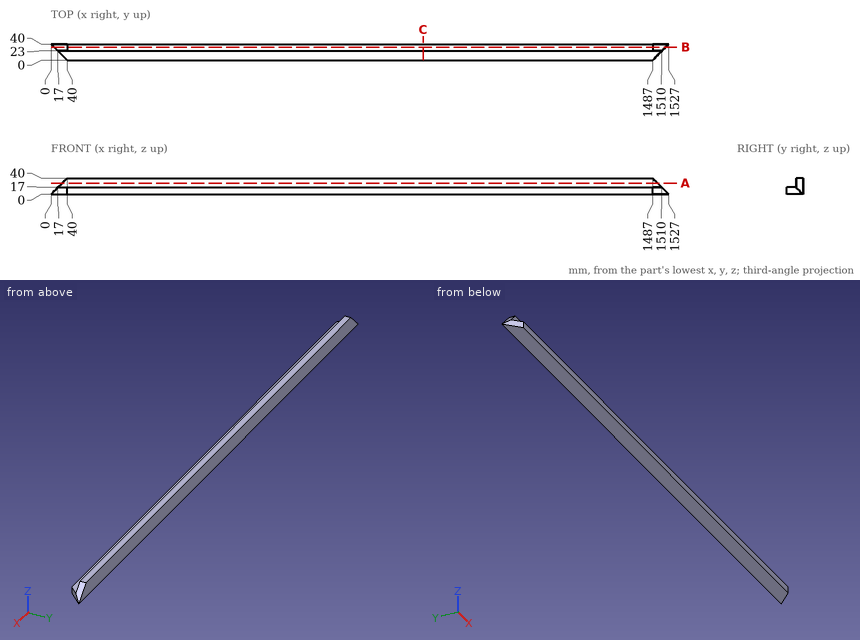
Check sheet for the drawn part. Datum: minimum x, y, z corner. Units: mm. Round coordinates to 2 decimals unless told otherwise and drop trailing zeros. Loops run counter-clockwise (first coordinate to the right, second up) from the corner with the lowest first, then second, coordinate; pieces in that order, holes last.
Item 1: Cross-section at B-B on y = 32.5. Record the boundary of the cut face in (x, z).
Item 2: Thickness scan on line 1 (Z direction, x = 881, y = 16); line 2 (Y direction, x = 729, z = 36); line 3 (X direction, y = 2, z = 7). Record the ranges inside material, lowest first.
Item 3: Cross-section at C-C on x = 919.5. Record the boundary of the cut face in (y, z), then the cut area to 3 significant figures.
Item 4: Cross-section at A-A on z = 28. Record the boundary of the cut face in (x, y).
Item 5: Gauge pin test, flat ends, axial feed: pin 1 (1 mm diameter, centred on y = 27.5, z = 8, fed in from -X); pin 2 (1 mm diameter, centred on y = 24, z = 34.5, fed in from +X); pin 3 (8 mm diameter, centred on x = 259, z = 22, fed in from -Y). Record the tip position at first contact, or that the pin passes through.
Answer sheet:
1. outline: (7.5, 0) - (1519.5, 0) - (1519.5, 7.5) - (1487, 40) - (40, 40) - (7.5, 7.5) - close
2. line 1: z = 0 to 17
2. line 2: y = 23 to 40
2. line 3: x = 38 to 1489
3. outline: (0, 0) - (40, 0) - (40, 40) - (23, 40) - (23, 17) - (0, 17) - close
3. area: 1,070 mm2
4. outline: (28, 23) - (1499, 23) - (1499, 40) - (28, 40) - close
5. pin 1: stops at x = 12
5. pin 2: stops at x = 1493
5. pin 3: stops at y = 23
